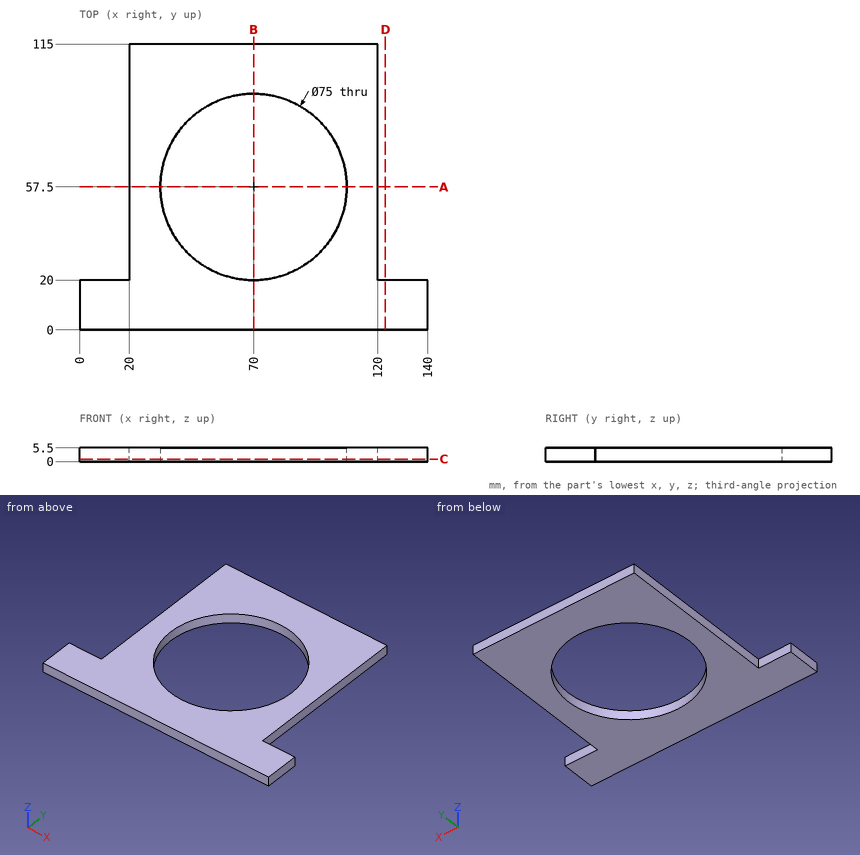
Drawing for the job (mm, zero at the part's lowest x, y, z). Coordinates: 2 decimals unless noted, no trailing zeros. Order: outer loops, then holes, each group sorted by start corner. A loop starts at its lowest first (then second) coordinate and runs counter-clockwise, first axis right, second up.
Item 1: Pin check, flat tips, straight feed: pin 1 Ø1.5 at (x, y) = (78.5, 22.5) entering from +Z; pin 2 Ø1.6 at (x, z) = (12, 2.5) entering from +Y; pin 3 Ø1.5 at (y, z) = (55, 3.5) entering from +X; pin 4 Ø1.6 at (y, z) = (79, 2.5) entering from -X. Stop position of each tip, or through.
Check sheet entries:
pin 1: passes through
pin 2: stops at y = 20
pin 3: stops at x = 120
pin 4: stops at x = 20
Item 2: Band-saw the part on B-B on x = 70. List the corners of the cut face in (y, z).
Check sheet entries:
outline: (0, 0) - (20, 0) - (20, 5.5) - (0, 5.5) - close; (95, 0) - (115, 0) - (115, 5.5) - (95, 5.5) - close
Item 3: Band-saw the part on A-A on y = 57.5. List the corners of the cut face in (x, z), plus the area to 4 significant figures.
Check sheet entries:
outline: (20, 0) - (32.5, 0) - (32.5, 5.5) - (20, 5.5) - close; (107.5, 0) - (120, 0) - (120, 5.5) - (107.5, 5.5) - close
area: 137.5 mm2
Item 4: Drill centre lines: L1, parallel to Y at x = 70, z = 4.1; L2, parallel to X at y = 57.5, z = 4.35; L3, parallel to Y at x = 37.5, z = 4.7. Where is each one in solid material? Low to high.
Check sheet entries:
L1: y = 0 to 20, 95 to 115
L2: x = 20 to 32.5, 107.5 to 120
L3: y = 0 to 38.79, 76.21 to 115
Item 5: Band-saw the part on D-D on x = 123. List the corners of the cut face in (y, z).
Check sheet entries:
outline: (0, 0) - (20, 0) - (20, 5.5) - (0, 5.5) - close
Item 6: Band-saw the part on C-C on z = 1. List the corners of the cut face in (x, y).
Check sheet entries:
outline: (0, 0) - (140, 0) - (140, 20) - (120, 20) - (120, 115) - (20, 115) - (20, 20) - (0, 20) - close; hole circle Ø75 at (70, 57.5)
